Can you work these out from the model? Positions are in its coordinate system, mm. Face numbers are marked on the shaded views. A direction names the side the tool comes from. Coordinates: 2 decimals unless noted, no trailing zeros. Order: outer loops, then holes, each group sorted by start corner. A loop starts at its lowest first (then second) coordinate and runs counter-clockwise, first axis right, second up. Notation, with made-up numbers: M 26.5,38 L 63.5,38 A19 ccw 63.5,73 Z; hole C 42.5,6 d2. An arc over 180 degrees is marked long. Answer as CSV lines item,"result". Start each with the question number.
1. I need wall thicknesses on line 1 along X through (y, z) = (10.5, 18) (3 decimals); line 2 along Z through (x, y) = (-5.5, -11.5); line 3 along Y through (x, z) = (-5, 15.75). Which ranges of each line are inside material? Lowest first, please. Write a range as from..to.
2. If we section it at C-C (z = -0.5): List the corners of the cut face in (x, y) for me.
3. If we section it at B-B (y = 0): List the corners of the cut face in (x, z) for me (3 decimals).
4. Will these pins go through, and if not, where does the flat tip stop? pin 1 (6 mm diameter, centred on y = -11.5, z = 5.5, fed in from -X); pin 2 (2 mm diameter, centred on y = -1, z = 9, fed in from +X) (3 decimals); pin 3 (2 mm diameter, centred on y = -4, z = 13, fed in from -X) (3 decimals).
5. If we section it at A-A (y = 5): List the corners of the cut face in (x, z) for me (3 decimals).
6. On a 3-axis mill with a long thin cutter (end or side, diameter ignored), from which of +Z, -Z, +X, -X, +Y, -Y can I reach the whole of each face in a straight line? I mean the marked faces 1 and 2. Say none if no direction works.
7. If we mould it in two halves opening along Z, with no side actions, what happens to the marked faces 3, 4, 5 and 6? For each: released by +Z, released by -Z, zero draft, split by the parting line, or undercut.
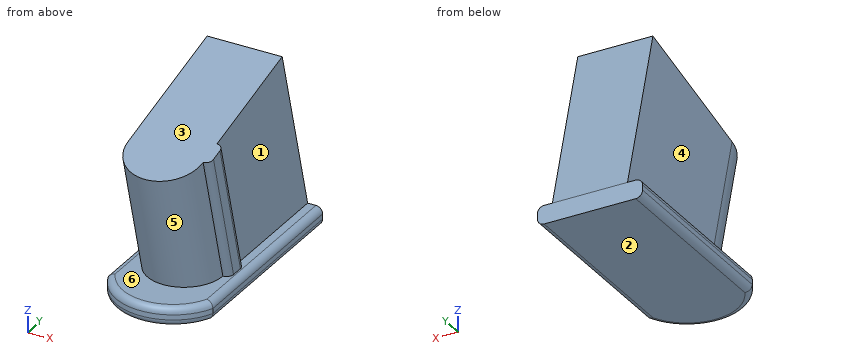
```python
from build123d import *

# Parameters (mm, degrees)
F2_W         = 1
F2_H         = 3.75
F3_DEPTH     = 20
F0_W         = 11.15
F0_H         = 22.225
F0_H_2       = 6.0527027428
F4_DEPTH     = 25
F5_DEPTH     = 2.75
F6_T1_DEPTH  = 33.7778691508
F6_T4_ANGLE  = 166.9020242579
F6_T6_ANGLE  = 166.9020242579
F6_T10_DEPTH = 25
F6_T15_DEPTH = 26.0048094716


# Not quite as in the source:
# - a fillet or chamfer that OpenCascade refuses, or shapes differently, is made with other operations: its cross-section is extruded or revolved along the edge and cut away or added


with BuildPart() as f3:
    # F2 (on line) → F3 (new body, symmetric)
    with BuildSketch(Plane(origin=(0, -0.3533579975, 1.31875), x_dir=(1, 0, 0), z_dir=(0, 0.2588190451, -0.9659258263))):
        with BuildLine():
            ThreePointArc((5.575, 5.0952587337), (0, 10.6702587337), (-5.575, 5.0952587337))
            Line((-5.575, 5.0952587337), (5.575, 5.0952587337))
        make_face()
        Polygon((5.575, 5.0952587337), (-5.575, 5.0952587337), (-5.575, -16.3724427556), (5.575, -16.3724427556), (5.575, 1.3452587337), align=None)
        with Locations((6.075, 3.2202587337)):
            Rectangle(F2_W, F2_H)
    extrude(amount=F3_DEPTH, both=True)

    # F0 (on Top) → F4 (cut)
    with BuildSketch(Plane.XY):
        with BuildLine():
            Line((5.575, -5.275), (-5.575, -5.275))
            ThreePointArc((-5.575, -5.275), (0, -10.85), (5.575, -5.275))
        make_face()
        with BuildLine():
            Line((-5.575, 16.95), (-7.8, 16.95))
            Line((-7.8, 16.95), (-7.8, -11.8278691508))
            ThreePointArc((-7.8, -11.8278691508), (-4.6657321086, -15.5549942921), (0, -16.95))
            ThreePointArc((0, -16.95), (4.6657321086, -15.5549942921), (7.8, -11.8278691508))
            Line((7.8, -11.8278691508), (7.8, 16.95))
            Line((7.8, 16.95), (5.575, 16.95))
            Line((5.575, 16.95), (5.575, -5.275))
            ThreePointArc((5.575, -5.275), (0, -10.85), (-5.575, -5.275))
            Line((-5.575, -5.275), (-5.575, 16.95))
        make_face()
        with Locations((0, 5.8375)):
            Rectangle(F0_W, F0_H)
        with Locations((0, 19.9763513714)):
            Rectangle(F0_W, F0_H_2)
    extrude(amount=-F4_DEPTH, mode=Mode.SUBTRACT)

    # F0 (on Top) → F5 (join)
    with BuildSketch(Plane.XY):
        with BuildLine():
            Line((-5.575, 16.95), (-7.8, 16.95))
            Line((-7.8, 16.95), (-7.8, -11.8278691508))
            ThreePointArc((-7.8, -11.8278691508), (-4.6657321086, -15.5549942921), (0, -16.95))
            ThreePointArc((0, -16.95), (4.6657321086, -15.5549942921), (7.8, -11.8278691508))
            Line((7.8, -11.8278691508), (7.8, 16.95))
            Line((7.8, 16.95), (5.575, 16.95))
            Line((5.575, 16.95), (5.575, -5.275))
            ThreePointArc((5.575, -5.275), (0, -10.85), (-5.575, -5.275))
            Line((-5.575, -5.275), (-5.575, 16.95))
        make_face()
        with BuildLine():
            Line((5.575, -5.275), (-5.575, -5.275))
            ThreePointArc((-5.575, -5.275), (0, -10.85), (5.575, -5.275))
        make_face()
        with Locations((0, 5.8375)):
            Rectangle(F0_W, F0_H)
    extrude(amount=-F5_DEPTH)

    # F6: fillet of radius 1 on 8 edges, made by hand

    # F6_s2 → F6_t1 (cut)
    with BuildSketch(Plane.XZ.offset(-19.45)):
        with BuildLine():
            ThreePointArc((6.8, 0), (7.5071067812, -0.2928932188), (7.8, -1))
            Line((7.8, -1), (7.8, 0))
            Line((7.8, 0), (6.8, 0))
        make_face()
        with BuildLine():
            ThreePointArc((6.8, -2.75), (7.5071067812, -2.4571067812), (7.8, -1.75))
            Line((7.8, -1.75), (7.8, -2.75))
            Line((7.8, -2.75), (6.8, -2.75))
        make_face()
        with BuildLine():
            ThreePointArc((-7.8, -1), (-7.5071067812, -0.2928932188), (-6.8, 0))
            Line((-6.8, 0), (-7.8, 0))
            Line((-7.8, 0), (-7.8, -1))
        make_face()
        with BuildLine():
            ThreePointArc((-7.8, -1.75), (-7.5071067812, -2.4571067812), (-6.8, -2.75))
            Line((-6.8, -2.75), (-7.8, -2.75))
            Line((-7.8, -2.75), (-7.8, -1.75))
        make_face()
    extrude(amount=F6_T1_DEPTH, mode=Mode.SUBTRACT)

    # F6_s3 → F6_t4 (revolve, cut)
    with BuildSketch(Plane(origin=(0.9574563888, -8.3400822912, 0), x_dir=(0, 0, 1), z_dir=(-0.1140526759, 0.9934747038, 0))):
        with BuildLine():
            ThreePointArc((-1, -9.4637451111), (-0.2928932188, -9.1708518923), (0, -8.4637451111))
            Line((0, -8.4637451111), (0, -9.4637451111))
            Line((0, -9.4637451111), (-1, -9.4637451111))
        make_face()
    revolve(axis=Axis((0, -8.45, 0), (0, 0, 1)), revolution_arc=F6_T4_ANGLE, mode=Mode.SUBTRACT)

    # F6_s5 → F6_t6 (revolve, cut)
    with BuildSketch(Plane(origin=(0.9574563888, -8.3400822912, 0), x_dir=(0, 0, 1), z_dir=(-0.1140526759, 0.9934747038, 0))):
        with BuildLine():
            ThreePointArc((-1.75, -9.4637451111), (-2.4571067812, -9.1708518923), (-2.75, -8.4637451111))
            Line((-2.75, -8.4637451111), (-2.75, -9.4637451111))
            Line((-2.75, -9.4637451111), (-1.75, -9.4637451111))
        make_face()
    revolve(axis=Axis((0, -8.45, -2.75), (0, 0, 1)), revolution_arc=F6_T6_ANGLE, mode=Mode.SUBTRACT)


with BuildPart() as f6_tool8:
    # F6_s9 → F6_t10 (new body)
    with BuildSketch(Plane(origin=(0, 0.2936896152, -1.0960645657), x_dir=(1, 0, 0), z_dir=(0, -0.2588190451, 0.9659258263))):
        with BuildLine():
            ThreePointArc((5.575, -5.0952587337), (6.2821067812, -4.8023655149), (6.575, -4.0952587337))
            Line((6.575, -4.0952587337), (6.575, -5.0952587337))
            Line((6.575, -5.0952587337), (5.575, -5.0952587337))
        make_face()
    extrude(amount=F6_T10_DEPTH)

    split(bisect_by=Plane.XY, keep=Keep.TOP)


with BuildPart() as f3_1:
    add(f3.part)

    # F6_t7: cut F6_tool8
    add(f6_tool8.part, mode=Mode.SUBTRACT)


with BuildPart() as f6_tool13:
    # F6_s14 → F6_t15 (new body)
    with BuildSketch(Plane(origin=(0, 0.5537534432, -2.0666359849), x_dir=(1, 0, 0), z_dir=(0, -0.2588190451, 0.9659258263))):
        with BuildLine():
            ThreePointArc((6.575, -2.3452587337), (6.2821067812, -1.6381519525), (5.575, -1.3452587337))
            Line((5.575, -1.3452587337), (6.575, -1.3452587337))
            Line((6.575, -1.3452587337), (6.575, -2.3452587337))
        make_face()
    extrude(amount=F6_T15_DEPTH)

    split(bisect_by=Plane.XY, keep=Keep.TOP)


with BuildPart() as f3_2:
    add(f3_1.part)

    # F6_t12: cut F6_tool13
    add(f6_tool13.part, mode=Mode.SUBTRACT)


solid = f3_2.part
```
Solved:
1,line 1,"-5.575..5.575"
1,line 2,"-2.75..0"
1,line 3,"-12.05..12.73"
2,outline,"M -7.67,-11.8 A8.37 ccw 7.67,-11.8 L 7.67,16.95 L -7.67,16.95 Z"
3,outline,"M -7.8,-1.75 A1 ccw -6.8,-2.75 L 6.8,-2.75 A1 ccw 7.8,-1.75 L 7.8,-1 A1 ccw 6.8,0 L 5.575,0 L 5.575,22.119 L -5.575,22.119 L -5.575,0 L -6.8,0 A1 ccw -7.8,-1 Z"
4,pin 1,"x = -5.34"
4,pin 2,"x = 5.575"
4,pin 3,"x = -5.575"
5,outline,"M -7.8,-1.75 A1 ccw -6.8,-2.75 L 6.8,-2.75 A1 ccw 7.8,-1.75 L 7.8,-1 A1 ccw 6.8,0 L 5.575,0 L 5.575,23.459 L -5.575,23.459 L -5.575,0 L -6.8,0 A1 ccw -7.8,-1 Z"
6,face 1,"+Z, +X, +Y"
6,face 2,"-Z, +X, -X, +Y, -Y"
7,face 3,"released by +Z"
7,face 4,"zero draft"
7,face 5,"undercut"
7,face 6,"undercut"
